Can you work these out from the drawing? Everything is in mm from the part's minimum corner. Coordinates: 2 decimals unless noted, no trailing zeros. Write each loop counter-clockwise with the first axis right and the second up, starting at its lowest first coordinate (ties: lowest second). Pieces come first, ordered by that corner, then holes.
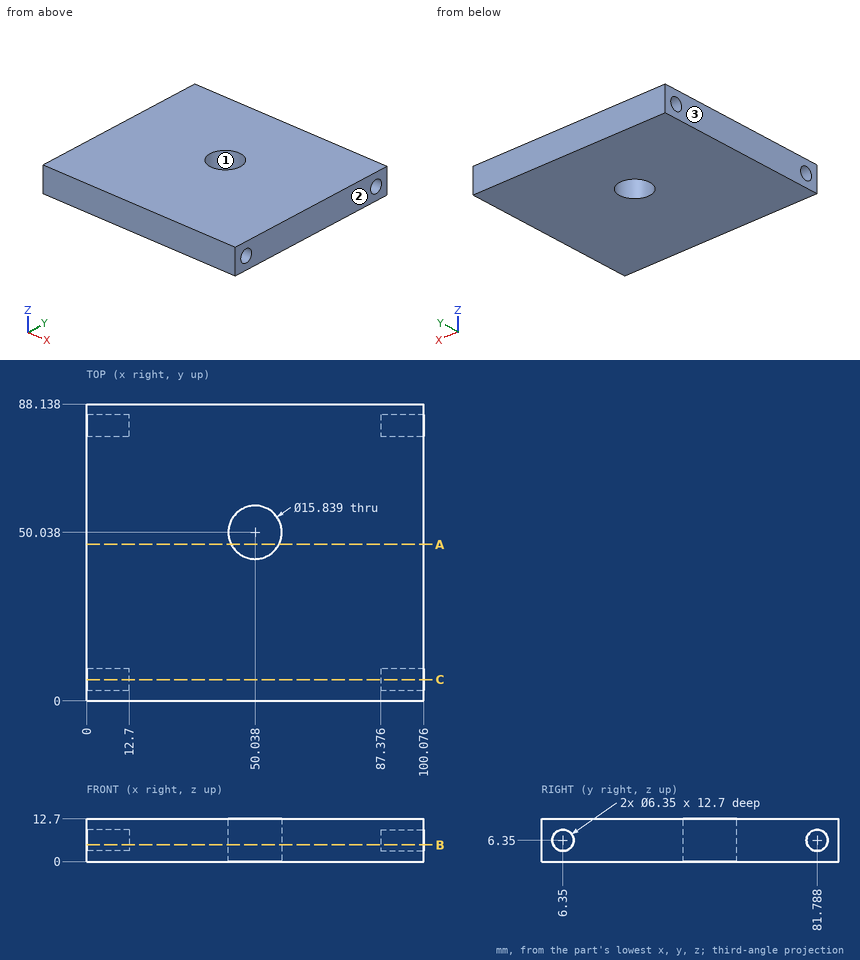
1. For pin 1 Ø5 at (y, z) = (6.35, 6.35) entering from -X; pin 2 Ø3 at (y, z) = (6, 5) entering from +X; pin 3 Ø14.5 at (x, y) = (50.038, 50.038) entering from -Z, each with a flat end and sliding along its axis, tell me the tip position at first contact or that it passes through.
2. If I drill on line 1 (Y direction, x = 93, z = 6.5); line 2 (Z direction, x = 4, y = 6) (1 decimal); line 3 (X direction, y = 6.5, z = 6), over which ranges is the centre line in solid material (lowest first)?
3. I want a section at A-A (y = 46.5). List the corners of the cut face in (x, z) for me, then the cut area to 3 significant figures.
4. I want a section at B-B (z = 5). List the corners of the cut face in (x, y) for me (1 decimal), then the cut area to 3 significant figures.
5. Thinking about a two-plate mould opening in X: for the marked faces 1, 2 and 3, which applies, pulls with the +X half, pulls with the -X half, needs draft (parallel to the pull), parting line crosses it, or undercut?
6. I want a section at C-C (y = 6.35). List the corners of the cut face in (x, z) for me (1 decimal), then the cut area to 3 significant figures.
Response values:
1. pin 1: stops at x = 12.7
1. pin 2: stops at x = 87.38
1. pin 3: passes through
2. line 1: y = 0 to 3.18, 9.52 to 78.62, 84.96 to 88.14
2. line 2: z = 0 to 3.2, 9.5 to 12.7
2. line 3: x = 12.7 to 87.38
3. outline: (0, 0) - (42.95, 0) - (42.95, 12.7) - (0, 12.7) - close; (57.12, 0) - (100.08, 0) - (100.08, 12.7) - (57.12, 12.7) - close
3. area: 1,090 mm2
4. outline: (0, 0) - (100.1, 0) - (100.1, 3.5) - (87.4, 3.5) - (87.4, 9.2) - (100.1, 9.2) - (100.1, 78.9) - (87.4, 78.9) - (87.4, 84.7) - (100.1, 84.7) - (100.1, 88.1) - (0, 88.1) - (0, 84.7) - (12.7, 84.7) - (12.7, 78.9) - (0, 78.9) - (0, 9.2) - (12.7, 9.2) - (12.7, 3.5) - (0, 3.5) - close; hole circle Ø15.8 at (50, 50)
4. area: 8,330 mm2
5. face 1: undercut
5. face 2: pulls with the +X half
5. face 3: pulls with the -X half
6. outline: (0, 0) - (100.1, 0) - (100.1, 3.2) - (87.4, 3.2) - (87.4, 9.5) - (100.1, 9.5) - (100.1, 12.7) - (0, 12.7) - (0, 9.5) - (12.7, 9.5) - (12.7, 3.2) - (0, 3.2) - close
6. area: 1,110 mm2
